```python
from build123d import *

# Parameters (mm, degrees)
SKETCH1_R           = 1.2499975
BOSS_EXTRUDE1_DEPTH = 1.999996
SKETCH2_W           = 5.0038
SKETCH2_H           = 22.6000056
BOSS_EXTRUDE2_DEPTH = 25.0000008


with BuildPart() as part:
    # Sketch1 → Boss-Extrude1 (new body)
    with BuildSketch(Plane(origin=(0, 0, 0), x_dir=(1, 0, 0), z_dir=(0, 1, 0))):
        with BuildLine():
            Line((-10.494133055, 1.188533953), (10.505875745, 1.188533953))
            ThreePointArc((10.505875745, 1.188533953), (12.380878345, -0.686468647), (10.505875745, -2.561471247))
            Line((10.505875745, -2.561471247), (-10.494133055, -2.561471247))
            ThreePointArc((-10.494133055, -2.561471247), (-12.369135655, -0.686468647), (-10.494133055, 1.188533953))
        make_face()
        with Locations(Location((-8.744123855, -0.686468647, 0), (0, 0, 270))):
            Circle(SKETCH1_R, mode=Mode.SUBTRACT)
        with Locations(Location((8.755866545, -0.686468647, 0), (0, 0, 90))):
            Circle(SKETCH1_R, mode=Mode.SUBTRACT)
    extrude(amount=BOSS_EXTRUDE1_DEPTH)

    # Sketch2 → Boss-Extrude2 (add)
    with BuildSketch(Plane.XZ):
        with Locations((-7.992233055, 13.861474047)):
            Rectangle(SKETCH2_W, SKETCH2_H)
    extrude(amount=-BOSS_EXTRUDE2_DEPTH)


solid = part.part
```
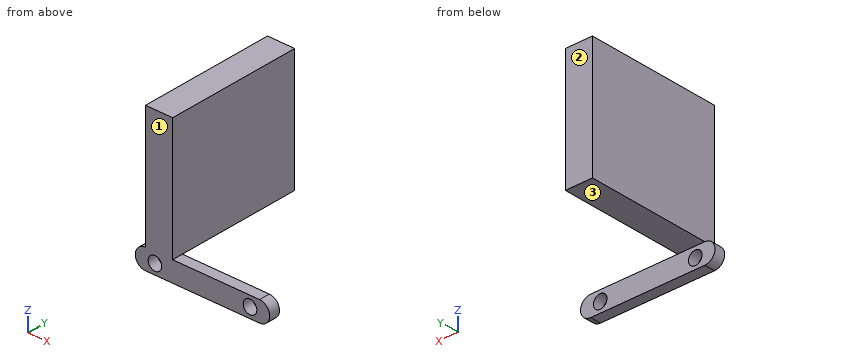
Could you check a few things on this model? Use its own coordinates, in mm. Face numbers are marked on the shaded views. Give positions to 0.01 mm unless a question says otherwise; leave off trailing zeros. Loops run counter-clockwise (first coordinate to the right, second up) from the corner with the lowest first, then second, coordinate; pieces in that order, holes last. Notation, with made-up numbers: (-24.5, 81.5) - (-3.5, 81.5) arc R14 cw to (-3.5, 98.5) - close; hole circle Ø4 at (-7.75, 27.5). An arc over 180 degrees is marked (long way). Answer in a Markdown table with one row per item. Add a question column.
Q1. We'd pull the mould along Y, two halves only. Please class the marked faces 1, 2 and 3: +Y half, -Y half, draft (parallel to the pull), parting line (faces both ways), or undercut.
Q2. For pin 1 (2.5 mm diameter, centred on x = -7, y = 16.5, fed in from -Z); pin 2 (5 mm diameter, centred on y = 21.5, z = 13, fed in from -X); pin 3 (1 mm diameter, centred on x = 6, y = 1.5, fed in from +Z), each with a flat end and sliding along its axis, tell me the tip position at first contact or that it passes through.
Q3. If we section it at A-A (x = -8): List the corners of the cut face in (y, z) for me.
Q4. If we section it at C-C (y = 14.5): List the corners of the cut face in (x, z) for me.
Q5. If we section it at B-B (z = 17): List the corners of the cut face in (x, y) for me.
Q6. Please list where these lines run through material, in increasing order: L1, parallel to X at y = 11.75, z = 21.5; L2, parallel to Z at x = -9, y = 10.75; L3, parallel to Y at x = 5.5, z = 1. Write a range as from..to.
The answers:
| question | item | result |
|---|---|---|
| 1 | face 1 | -Y half |
| 1 | face 2 | +Y half |
| 1 | face 3 | draft |
| 2 | pin 1 | stops at z = 2.56 |
| 2 | pin 2 | stops at x = -10.49 |
| 2 | pin 3 | stops at z = 2.56 |
| 3 | outline | (0, -1.19) - (2, -1.19) - (2, -0.32) - (0, -0.32) - close; (0, 1.69) - (2, 1.69) - (2, 2.56) - (25, 2.56) - (25, 25.16) - (0, 25.16) - close |
| 4 | outline | (-10.49, 2.56) - (-5.49, 2.56) - (-5.49, 25.16) - (-10.49, 25.16) - close |
| 5 | outline | (-10.49, 0) - (-5.49, 0) - (-5.49, 25) - (-10.49, 25) - close |
| 6 | L1 | x = -10.49..-5.49 |
| 6 | L2 | z = 2.56..25.16 |
| 6 | L3 | y = 0..2 |
